Build history of the part. All positions in model axes, mm. Give positions to 0.01 mm unless a question says otherwise; leave off trailing zeros. Order: outer loops, then holes, each group sorted by start corner. A loop starts at its lowest first (then second) coordinate and runs counter-clockwise, first axis right, second up. Notation, with made-up numbers: (55, -26) - (81, -26) arc R28 cw to (81, 12) - close; hole circle Ø3 at (71, -14). An arc over 180 degrees is marked (long way). Use a Markdown table: item, result. Add a question column.
(1) Slice it at C-C (y = -178). Write the cut outline in (x, z), then the cut area to 3 significant figures.
(2) Wall check: line 1 (Y direction, x = -190, z = 20.25); line 2 (X direction, y = -137, z = 30.5); line 3 (Y direction, x = -285.75, z = 8.75). Give the ranges that are in metal, low to high.
(3) Slice it at D-D (y = 8). Write the cut outline in (x, z), then the cut area to 3 significant figures.
(4) Flat gauge pins, fed straight in: pin 1 (6.5 mm diameter, centred on y = 142.5, z = 34, fed in from +X); pin 2 (19 mm diameter, centred on x = 196, y = -154.5, fed in from +Z); pin 3 (4 mm diameter, centred on y = 139, z = 33, fed in from -X). Where does each tip first touch, or does it go through?
(5) Slice it at A-A (y = 87). Write the cut outline in (x, z), then the cut area to 3 significant figures.
(6) Slice it at B-B (z = 9.5). Count the separate pieces of the cut face and the enclosed holes in it, then the cut area to 3 significant figures.
from build123d import *

# Parameters (mm, degrees)
F0_R     = 4
F1_DEPTH = 38.1
F2_R     = 5
F3_W     = 38.1
F3_H     = 88.9
F3_R     = 4
F4_DEPTH = 12.75
F5_R     = 5


with BuildPart() as f1:
    # F0 (on Top) → F1 (new body)
    with BuildSketch(Plane.XY):
        Polygon((253.5, 253.5), (-253.5, 253.5), (-253.5, 69.85), (-330.2, 69.85), (-330.2, -69.85), (-253.5, -69.85), (-253.5, -253.5), (253.5, -253.5), (253.5, -69.85), (330.2, -69.85), (330.2, 69.85), (253.5, 69.85), align=None)
        with Locations((-190, -190)):
            Circle(F0_R, mode=Mode.SUBTRACT)
        with Locations((-190, -126.5)):
            Circle(F0_R, mode=Mode.SUBTRACT)
        with Locations((-285.75, -25.4)):
            Circle(F0_R, mode=Mode.SUBTRACT)
        with Locations((190, -190)):
            Circle(F0_R, mode=Mode.SUBTRACT)
        with Locations((190, -126.5)):
            Circle(F0_R, mode=Mode.SUBTRACT)
        with Locations((285.75, -25.4)):
            Circle(F0_R, mode=Mode.SUBTRACT)
        with Locations((-285.75, 25.4)):
            Circle(F0_R, mode=Mode.SUBTRACT)
        with Locations((-190, 126.5)):
            Circle(F0_R, mode=Mode.SUBTRACT)
        with Locations((-190, 190)):
            Circle(F0_R, mode=Mode.SUBTRACT)
        with Locations((285.75, 25.4)):
            Circle(F0_R, mode=Mode.SUBTRACT)
        with Locations((190, 126.5)):
            Circle(F0_R, mode=Mode.SUBTRACT)
        with Locations((190, 190)):
            Circle(F0_R, mode=Mode.SUBTRACT)
    extrude(amount=F1_DEPTH)

    # F2
    f2_edges = [f1.edges().sort_by_distance(p)[0] for p in [
        (0, -253.5, 38.1),
        (-253.5, -161.675, 38.1),
        (-253.5, -253.5, 19.05),
        (-253.5, -69.85, 19.05),
        (-291.85, -69.85, 38.1),
        (-330.2, -69.85, 19.05),
        (-330.2, 0, 38.1),
        (-291.85, 69.85, 38.1),
        (-253.5, 161.675, 38.1),
        (0, 253.5, 38.1),
        (253.5, 161.675, 38.1),
        (291.85, 69.85, 38.1),
        (253.5, 69.85, 19.05),
        (253.5, 253.5, 19.05),
        (-253.5, 253.5, 19.05),
        (-253.5, 69.85, 19.05),
        (-330.2, 69.85, 19.05),
        (291.85, -69.85, 38.1),
        (330.2, 0, 38.1),
        (330.2, 69.85, 19.05),
        (330.2, -69.85, 19.05),
        (253.5, -69.85, 19.05),
        (253.5, -161.675, 38.1),
        (253.5, -253.5, 19.05),
    ]]
    fillet(f2_edges, radius=F2_R)

    # F3 (on face) → F4 (cut)
    with BuildSketch(Plane.XY.offset(38.1)):
        with Locations((-190, 158.25)):
            Rectangle(F3_W, F3_H)
        with Locations((-190, 126.5)):
            Circle(F3_R, mode=Mode.SUBTRACT)
        with Locations((-190, 190)):
            Circle(F3_R, mode=Mode.SUBTRACT)
        with Locations((190, 158.25)):
            Rectangle(F3_W, F3_H)
        with Locations((190, 126.5)):
            Circle(F3_R, mode=Mode.SUBTRACT)
        with Locations((190, 190)):
            Circle(F3_R, mode=Mode.SUBTRACT)
        with Locations((285.75, 0)):
            Rectangle(F3_W, F3_H)
        with Locations((285.75, -25.4)):
            Circle(F3_R, mode=Mode.SUBTRACT)
        with Locations((285.75, 25.4)):
            Circle(F3_R, mode=Mode.SUBTRACT)
        with Locations((190, -158.25)):
            Rectangle(F3_W, F3_H)
        with Locations((190, -190)):
            Circle(F3_R, mode=Mode.SUBTRACT)
        with Locations((190, -126.5)):
            Circle(F3_R, mode=Mode.SUBTRACT)
        with Locations((-190, -158.25)):
            Rectangle(F3_W, F3_H)
        with Locations((-190, -190)):
            Circle(F3_R, mode=Mode.SUBTRACT)
        with Locations((-190, -126.5)):
            Circle(F3_R, mode=Mode.SUBTRACT)
        with Locations((-285.75, 0)):
            Rectangle(F3_W, F3_H)
        with Locations((-285.75, -25.4)):
            Circle(F3_R, mode=Mode.SUBTRACT)
        with Locations((-285.75, 25.4)):
            Circle(F3_R, mode=Mode.SUBTRACT)
    extrude(amount=-F4_DEPTH, mode=Mode.SUBTRACT)

    # F5
    f5_edges = [f1.edges().sort_by_distance(p)[0] for p in [
        (170.95, 202.7, 31.725),
        (170.95, 113.8, 31.725),
        (209.05, 202.7, 31.725),
        (209.05, 113.8, 31.725),
        (304.8, -44.45, 31.725),
        (304.8, 44.45, 31.725),
        (266.7, 44.45, 31.725),
        (266.7, -44.45, 31.725),
        (170.95, -202.7, 31.725),
        (170.95, -113.8, 31.725),
        (209.05, -113.8, 31.725),
        (209.05, -202.7, 31.725),
        (-209.05, -113.8, 31.725),
        (-170.95, -113.8, 31.725),
        (-170.95, -202.7, 31.725),
        (-209.05, -202.7, 31.725),
        (-304.8, -44.45, 31.725),
        (-266.7, -44.45, 31.725),
        (-266.7, 44.45, 31.725),
        (-304.8, 44.45, 31.725),
        (-209.05, 202.7, 31.725),
        (-170.95, 202.7, 31.725),
        (-170.95, 113.8, 31.725),
        (-209.05, 113.8, 31.725),
    ]]
    fillet(f5_edges, radius=F5_R)


solid = f1.part
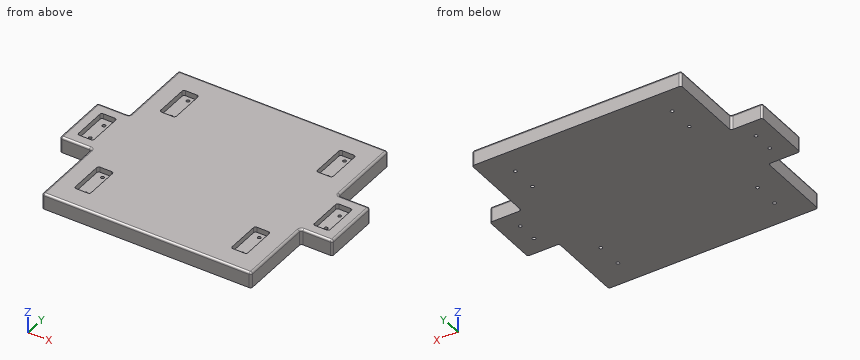
Solution:
| question | item | result |
|---|---|---|
| 1 | outline | (-253.5, 0) - (253.5, 0) - (253.5, 33.1) arc R5 ccw to (248.5, 38.1) - (209.05, 38.1) - (209.05, 25.35) - (170.95, 25.35) - (170.95, 38.1) - (-170.95, 38.1) - (-170.95, 25.35) - (-209.05, 25.35) - (-209.05, 38.1) - (-248.5, 38.1) arc R5 ccw to (-253.5, 33.1) - close |
| 1 | area | 18,300 mm2 |
| 2 | line 1 | -253.5 to -194, -186 to -130.5, -122.5 to 122.5, 130.5 to 186, 194 to 253.5 |
| 2 | line 2 | -253.5 to -209.05, -170.95 to 170.95, 209.05 to 253.5 |
| 2 | line 3 | -69.85 to -29.4, -21.4 to 21.4, 29.4 to 69.85 |
| 3 | outline | (-330.2, 0) - (330.2, 0) - (330.2, 33.1) arc R5 ccw to (325.2, 38.1) - (304.8, 38.1) - (304.8, 25.35) - (266.7, 25.35) - (266.7, 38.1) - (-266.7, 38.1) - (-266.7, 25.35) - (-304.8, 25.35) - (-304.8, 38.1) - (-325.2, 38.1) arc R5 ccw to (-330.2, 33.1) - close |
| 3 | area | 24,200 mm2 |
| 4 | pin 1 | x = 253.5 |
| 4 | pin 2 | z = 25.35 |
| 4 | pin 3 | x = -253.5 |
| 5 | outline | (-253.5, 0) - (253.5, 0) - (253.5, 33.1) arc R5 ccw to (248.5, 38.1) - (-248.5, 38.1) arc R5 ccw to (-253.5, 33.1) - close |
| 5 | area | 19,300 mm2 |
| 6 | separate pieces | 1 |
| 6 | enclosed holes | 12 |
| 6 | area | 278,000 mm2 |
